Work out the finished part from the listing and answer in its coordinate system (mm). A direction names the side the tool comes from. Round coordinates to 2 decimals unless told otherwise and drop trailing zeros. Write each loop counter-clockwise with the first axis right and the second up, starting at its lowest first coordinate (ties: lowest second). Pieces come first, ordered by that corner, then holes. Notation, with made-up numbers: (48, -34) - (91, -34) arc R15 ccw to (91, -15) - close; hole circle Ø6 at (27, 26). An arc over 180 degrees is marked (long way). Write item = value, one per line. Start each with the question number.
from build123d import *

# Parameters (mm, degrees)
F1_DEPTH = 7.62
F2_T     = -2.54


with BuildPart() as f1:
    # F0 (on Front) → F1 (new body)
    with BuildSketch(Plane.XZ):
        with BuildLine():
            Line((59.459757, 60.312882), (-60.681279, 60.312882))
            ThreePointArc((-60.681279, 60.312882), (-65.171407, 58.45301), (-67.031279, 53.962882))
            Line((-67.031279, 53.962882), (-67.031279, -55.184408))
            ThreePointArc((-67.031279, -55.184408), (-65.171407, -59.674537), (-60.681279, -61.534408))
            Line((-60.681279, -61.534408), (59.459757, -61.534408))
            ThreePointArc((59.459757, -61.534408), (63.949885, -59.674537), (65.809757, -55.184408))
            Line((65.809757, -55.184408), (65.809757, 53.962882))
            ThreePointArc((65.809757, 53.962882), (63.949885, 58.45301), (59.459757, 60.312882))
        make_face()
    extrude(amount=F1_DEPTH)

    # F2
    f2_openings = [f1.faces().sort_by_distance(p)[0] for p in [
        (-0.610761, -7.62, -0.610763),
    ]]
    offset(amount=F2_T, openings=f2_openings)


solid = f1.part
1. Find section C-C on x = 35. Give the vertices of the cut face in (y, z).
2. Find section A-A on y = -4.75. Give the vertices of the cut face in (x, z).
3. Which of the six approach directions +Z, -Z, +X, -X, +Y, -Y give full straight-line access (tool end or side, diameter ignored) to faces 5 (the face through (0, -4, 60.313)), 6 (the face through (-63.346, -5.044, 56.686))?
4. This flat-tipped pin is pushed along its axis until it touches: pin 1 (5 mm diameter, centred on x = -5.5, z = 3, fed in from -Y). Where does it stop, or does it pass through?
5. Find section B-B on z = -26.5. Give the vertices of the cut face in (x, y).
6. Consider line 1 (Z direction, x = -15, y = -5); line 2 (X direction, y = -4.5, z = 12); line 3 (Y direction, x = -34, z = -17.5). Determine where each line is inside the solid, lowest interval first.
7. For a pull along Z with two mould halves and no side action, classify faces 1 (the face through (-63.405, -5.044, -57.849)), 2 (the face through (63.9, -3.757, -59.724)), 3 (the face through (-2, -2.54, 0)), 4 (the face through (64, -3.8, 58.4)) as released by +Z, released by -Z, zero draft, split by the parting line, or undercut.
Answer key:
q1.outline = (-7.62, -61.53) - (0, -61.53) - (0, 60.31) - (-7.62, 60.31) - (-7.62, 57.77) - (-2.54, 57.77) - (-2.54, -58.99) - (-7.62, -58.99) - close
q2.outline = (-67.03, -55.18) arc R6.35 ccw to (-60.68, -61.53) - (59.46, -61.53) arc R6.35 ccw to (65.81, -55.18) - (65.81, 53.96) arc R6.35 ccw to (59.46, 60.31) - (-60.68, 60.31) arc R6.35 ccw to (-67.03, 53.96) - close; hole (-64.49, -55.18) arc R3.81 ccw to (-60.68, -58.99) - (59.46, -58.99) arc R3.81 ccw to (63.27, -55.18) - (63.27, 53.96) arc R3.81 ccw to (59.46, 57.77) - (-60.68, 57.77) arc R3.81 ccw to (-64.49, 53.96) - close
q3.face_5 = +Z, +X, -X, +Y, -Y
q3.face_6 = -Y
q4.pin_1 = -2.54
q5.outline = (-67.03, -7.62) - (-64.49, -7.62) - (-64.49, -2.54) - (63.27, -2.54) - (63.27, -7.62) - (65.81, -7.62) - (65.81, 0) - (-67.03, 0) - close
q6.line_1 = -61.53 to -58.99, 57.77 to 60.31
q6.line_2 = -67.03 to -64.49, 63.27 to 65.81
q6.line_3 = -2.54 to 0
q7.face_1 = undercut
q7.face_2 = released by -Z
q7.face_3 = undercut
q7.face_4 = released by +Z
